Input: part model. Units: mm. Frame: model coordinates. A direction names the side the tool comes from. Coordinates: 2 decimals unless noted, no trailing zeros. Loops run counter-clockwise (first coordinate to the right, second up) from the corner with the lowest first, then second, coordinate; pieces in that order, holes last. Notation, with made-up numbers: (-1.75, -20.5) -> (10.25, -20.5) arc R10 cw to (10.25, -16.5) -> close; hole circle Ø2 at (69, 13). An arc over 180 degrees is marked (long way). Put each result on its own line as item: value. Start each with the question number.
1) Cut plane A-A (x = -64). Return the cut outline in (y, z).
2) Cut plane C-C (x = -113). Return the cut outline in (y, z).
3) Cut plane B-B (y = 39.5). Return the cut outline in (x, z), plus the area to 3 significant figures.
4) Pull-direction query (Y, two-part tool) for faces 4 (the flat face through (-150, 164.261, 3)), 5 (the flat face through (-232, 122.261, 9)), 6 (the flat face through (-150, 17.261, 4)); classes: pulls with the +Y half, pulls with the -Y half, needs draft (parallel to the pull), parting line crosses it, or undercut.
5) Material intervals for L1, parallel to Y at x = -62, z = 7.75; L2, parallel to Y at x = -103, z = 9.5; L3, parallel to X at y = 86, z = 10.25, sorted ascending.
6) Set-up query: faces 1 (the flat face through (-232, 67.361, 9)), 2 (the flat face through (-232, 69.361, 9)), 3 (the flat face through (-109, 115.461, 9)). Return all of +Z, -Z, +X, -X, +Y, -Y with unobstructed straight access to the full face (end or side cutting, diameter ignored); none if empty.
7) Contact query for flat-ended pins moving along their axis: P1, Ø1.6, axis at y = 114, z = 8.5, coming from the -X side; P2, Ø4, axis at x = -65, z = 10.5, coming from the -Y side; P3, Ø2, axis at y = 105, z = 10.5, coming from the -X side. Output: stop coordinate, or through.
from build123d import *

# Parameters (mm, degrees)
SKETCH1_W           = 200
SKETCH1_H           = 150
BOSS_EXTRUDE1_DEPTH = 7
SKETCH2_W           = 13.6
SKETCH2_H           = 2
BOSS_EXTRUDE2_DEPTH = 5
SKETCH3_W           = 200
SKETCH3_H           = 7
CUT_EXTRUDE1_DEPTH  = 3


with BuildPart() as part:
    # Sketch1 → Boss-Extrude1 (new body)
    with BuildSketch(Plane.XY):
        with Locations((-148.719211823, 89.261083744)):
            Rectangle(SKETCH1_W, SKETCH1_H)
    extrude(amount=BOSS_EXTRUDE1_DEPTH)

    # Sketch2 → Boss-Extrude2 (add)
    with BuildSketch(Plane.XY.offset(7)):
        with Locations((-109.119211823, 114.461083744)):
            Rectangle(SKETCH2_W, SKETCH2_H)
        with Locations((-65.519211823, 104.961083744)):
            Rectangle(SKETCH2_W, SKETCH2_H)
        with Locations((-65.519211823, 123.261083744)):
            Rectangle(SKETCH2_W, SKETCH2_H)
        with Locations((-65.519211823, 86.661083744)):
            Rectangle(SKETCH2_W, SKETCH2_H)
        with Locations((-65.519211823, 68.361083744)):
            Rectangle(SKETCH2_W, SKETCH2_H)
        with Locations((-231.919211823, 104.961083744)):
            Rectangle(SKETCH2_W, SKETCH2_H)
        with Locations((-231.919211823, 123.261083744)):
            Rectangle(SKETCH2_W, SKETCH2_H)
        with Locations((-231.919211823, 86.661083744)):
            Rectangle(SKETCH2_W, SKETCH2_H)
        with Locations((-231.919211823, 68.361083744)):
            Rectangle(SKETCH2_W, SKETCH2_H)
        with Locations((-188.319211823, 114.461083744)):
            Rectangle(SKETCH2_W, SKETCH2_H)
        with Locations((-188.319211823, 77.861083744)):
            Rectangle(SKETCH2_W, SKETCH2_H)
        with Locations((-109.119211823, 77.861083744)):
            Rectangle(SKETCH2_W, SKETCH2_H)
    extrude(amount=BOSS_EXTRUDE2_DEPTH)

    # Sketch3 → Cut-Extrude1 (cut)
    with BuildSketch(Plane.XZ.offset(-14.261083744)):
        with Locations((-148.719211823, 3.5)):
            Rectangle(SKETCH3_W, SKETCH3_H)
    extrude(amount=-CUT_EXTRUDE1_DEPTH, mode=Mode.SUBTRACT)


solid = part.part
Results found:
1. outline: (17.26, 0) -> (164.26, 0) -> (164.26, 7) -> (124.26, 7) -> (124.26, 12) -> (122.26, 12) -> (122.26, 7) -> (105.96, 7) -> (105.96, 12) -> (103.96, 12) -> (103.96, 7) -> (87.66, 7) -> (87.66, 12) -> (85.66, 12) -> (85.66, 7) -> (69.36, 7) -> (69.36, 12) -> (67.36, 12) -> (67.36, 7) -> (17.26, 7) -> close
2. outline: (17.26, 0) -> (164.26, 0) -> (164.26, 7) -> (115.46, 7) -> (115.46, 12) -> (113.46, 12) -> (113.46, 7) -> (78.86, 7) -> (78.86, 12) -> (76.86, 12) -> (76.86, 7) -> (17.26, 7) -> close
3. outline: (-248.72, 0) -> (-48.72, 0) -> (-48.72, 7) -> (-248.72, 7) -> close
3. area: 1,400 mm2
4. face 4: pulls with the +Y half
4. face 5: undercut
4. face 6: pulls with the -Y half
5. L1: y = 67.36 to 69.36, 85.66 to 87.66, 103.96 to 105.96, 122.26 to 124.26
5. L2: y = 76.86 to 78.86, 113.46 to 115.46
5. L3: x = -238.72 to -225.12, -72.32 to -58.72
6. face 1: +Z, +X, -X, -Y
6. face 2: +Z, +X, -X
6. face 3: +Z, +X, -X, +Y
7. P1: stops at x = -195.12
7. P2: stops at y = 67.36
7. P3: stops at x = -238.72
